from build123d import *

# Parameters (mm, degrees)
SKETCH1_R           = 40.52203667
BOSS_EXTRUDE1_DEPTH = 20
FILLET1_R           = 45


with BuildPart() as part:
    # Sketch1 → Boss-Extrude1 (new body)
    with BuildSketch(Plane.XY):
        Polygon((-324.500042801, 0), (-36.61106831, 0), (-36.61106831, -72.630227613), (19.444444444, -30.98937664), (19.444444444, 0), (19.444444444, 300), (-180.555555556, 600), (-380.555555556, 300), (-380.555555556, 0), (-380.555555556, -30.98937664), (-324.500042801, -72.630227613), align=None)
        with Locations((-180.555555556, 199.47796333)):
            Circle(SKETCH1_R, mode=Mode.SUBTRACT)
        Polygon((-350.555555556, 98.955926659), (-307.046121917, 98.955926659), (-350.555555556, 40.384990781), align=None, mode=Mode.SUBTRACT)
        Polygon((-218.052993309, 18.381237109), (-277.907920592, 98.955926659), (-83.203190519, 98.955926659), (-143.058117802, 18.381237109), align=None, mode=Mode.SUBTRACT)
        Polygon((-40.212760909, 30), (-97.055418804, 30), (-68.634089856, 68.259836918), align=None, mode=Mode.SUBTRACT)
        Polygon((-350.555555556, 128.955926659), (-307.046121917, 128.955926659), (-307.046121917, 178.791030317), (-307.046121917, 221.457829656), (-307.046121917, 270), (-350.555555556, 270), (-350.555555556, 221.457829656), (-350.555555556, 178.791030317), align=None, mode=Mode.SUBTRACT)
        Polygon((-194.895952536, 524.406135398), (-246.308768225, 447.286911864), (-194.895952536, 447.286911864), align=None, mode=Mode.SUBTRACT)
        Polygon((-36.61106831, 330), (-96.633315679, 420.033371054), (-153.463987032, 330), align=None, mode=Mode.SUBTRACT)
        Polygon((-324.500042801, 330), (-207.64712408, 330), (-264.477795432, 420.033371054), align=None, mode=Mode.SUBTRACT)
        Polygon((-10.555555556, 40.384990781), (-54.064989194, 98.955926659), (-10.555555556, 98.955926659), align=None, mode=Mode.SUBTRACT)
        Polygon((-10.555555556, 128.955926659), (-10.555555556, 178.791030317), (-10.555555556, 221.457829656), (-10.555555556, 270), (-54.064989194, 270), (-54.064989194, 221.457829656), (-54.064989194, 178.791030317), (-54.064989194, 128.955926659), align=None, mode=Mode.SUBTRACT)
        Polygon((-320.898350202, 30), (-264.055692307, 30), (-292.477021255, 68.259836918), align=None, mode=Mode.SUBTRACT)
        with BuildLine():
            Line((-279.511482215, 270), (-279.511482215, 221.457829656))
            Line((-279.511482215, 221.457829656), (-247.564832021, 221.457829656))
            ThreePointArc((-247.564832021, 221.457829656), (-232.312774166, 247.379403578), (-207.64712408, 264.58867344))
            Line((-207.64712408, 264.58867344), (-207.64712408, 270))
            Line((-207.64712408, 270), (-279.511482215, 270))
        make_face(mode=Mode.SUBTRACT)
        with BuildLine():
            Line((-279.511482215, 128.955926659), (-279.511482215, 178.791030317))
            Line((-279.511482215, 178.791030317), (-247.975200012, 178.791030317))
            ThreePointArc((-247.975200012, 178.791030317), (-232.771073725, 152.076514844), (-207.64712408, 134.367253219))
            Line((-207.64712408, 134.367253219), (-207.64712408, 128.955926659))
            Line((-207.64712408, 128.955926659), (-279.511482215, 128.955926659))
        make_face(mode=Mode.SUBTRACT)
        with BuildLine():
            Line((-153.463987032, 134.367253219), (-153.463987032, 128.955926659))
            Line((-153.463987032, 128.955926659), (-81.599628896, 128.955926659))
            Line((-81.599628896, 128.955926659), (-81.599628896, 178.791030317))
            Line((-81.599628896, 178.791030317), (-113.135911099, 178.791030317))
            ThreePointArc((-113.135911099, 178.791030317), (-128.340037386, 152.076514844), (-153.463987032, 134.367253219))
        make_face(mode=Mode.SUBTRACT)
        with BuildLine():
            Line((-153.463987032, 264.58867344), (-153.463987032, 270))
            Line((-153.463987032, 270), (-81.599628896, 270))
            Line((-81.599628896, 270), (-81.599628896, 221.457829656))
            Line((-81.599628896, 221.457829656), (-113.54627909, 221.457829656))
            ThreePointArc((-113.54627909, 221.457829656), (-128.798336945, 247.379403578), (-153.463987032, 264.58867344))
        make_face(mode=Mode.SUBTRACT)
        Polygon((-114.802342886, 429.992241235), (-166.215158575, 429.992241235), (-166.215158575, 348.542048906), align=None, mode=Mode.SUBTRACT)
        Polygon((-114.802342886, 447.286911864), (-166.215158575, 524.406135398), (-166.215158575, 447.286911864), align=None, mode=Mode.SUBTRACT)
        Polygon((-246.308768225, 429.992241235), (-194.895952536, 348.542048906), (-194.895952536, 429.992241235), align=None, mode=Mode.SUBTRACT)
    extrude(amount=BOSS_EXTRUDE1_DEPTH)

    # Fillet1
    fillet1_edges = [part.edges().sort_by_distance(p)[0] for p in [
        (19.444444444, -30.98937664, 10),
        (-380.555555556, -30.98937664, 10),
        (-380.555555556, 300, 10),
        (-180.555555556, 600, 10),
        (19.444444444, 300, 10),
    ]]
    fillet(fillet1_edges, radius=FILLET1_R)


solid = part.part
CAD build for the part. Positions are in the model's coordinates, mm. A direction names the side the tool comes from. Give positions to 0.01 mm unless a question says otherwise; leave off trailing zeros. Loops run counter-clockwise (first coordinate to the right, second up) from the corner with the lowest first, then second, coordinate; pieces in that order, holes last. Notation, with made-up numbers: M 83,17 L 90,17 A27 ccw 90,54 Z; hole C -17,-2.75 d4. An arc over 180 degrees is marked long. Write each question's results on one line, items separated by ' | '.
Q1. Mould opens along Y. For faces 3 (the face through (-36.611, -36, 10)), 4 (the face through (-181.17, 563.87, 10.14)), 5 (the face through (-140.15, 485.31, 9.86)) say: pulls with the +Y half, pulls with the -Y half, needs draft (parallel to the pull), parting line crosses it, or undercut.
Geometry check:
face 3: needs draft | face 4: pulls with the +Y half | face 5: undercut
Q2. Band-saw the part on D-D on z = 7.5. Give the number of separate pieces and of enclosed holes in the cut face, and give its area (3 significant figures).
Geometry check:
separate pieces: 1 | enclosed holes: 18 | area: 123,000 mm²
Q3. Band-saw the part on B-B on x = -338. Write the cut outline in (y, z).
Geometry check:
outline: M -62.6,0 L 57.29,0 L 57.29,20 L -62.6,20 Z; M 98.96,0 L 128.96,0 L 128.96,20 L 98.96,20 Z; M 270,0 L 363.83,0 L 363.83,20 L 270,20 Z
Q4. Band-saw the part on A-A on y = 209. Write the cut outline in (x, z).
Geometry check:
outline: M -380.56,0 L -350.56,0 L -350.56,20 L -380.56,20 Z; M -307.05,0 L -219.94,0 L -219.94,20 L -307.05,20 Z; M -141.17,0 L -54.06,0 L -54.06,20 L -141.17,20 Z; M -10.56,0 L 19.44,0 L 19.44,20 L -10.56,20 Z
Q5. Flat gauge pins, fed straight in: P1, Ø8, axis at x = -188.5, y = 493.5, coming from the -Z side; P2, Ø10, axis at y = 361.5, z = 9, coming from the -X side; P3, Ø2, axis at x = -224.5, z = 3.5, coming from the +Y side; P4, Ø10, axis at y = 497, z = 10, coming from the -X side. Where does each tip first touch, or does it go through?
Geometry check:
P1: stops at z = 0 | P2: stops at x = -342.89 | P3: stops at y = 535.58 | P4: stops at x = -252.56
Q6. Which spindle directions (+Z, -Z, +X, -X, +Y, -Y) get a long thin tool onto all of the face, cutting with end or side? Do faces 1 (the face through (-380.556, 141, 10)), 2 (the face through (-81.6, 246, 10)). Say none if no direction does.
Geometry check:
face 1: +Z, -Z, -X, +Y, -Y | face 2: +Z, -Z
Q7. Band-saw the part on C-C on y = 372. Write the cut outline in (x, z), and give its area (3 significant figures).
Geometry check:
outline: M -332.56,0 L -296.5,0 L -296.5,20 L -332.56,20 Z; M -234.16,0 L -209.7,0 L -209.7,20 L -234.16,20 Z; M -194.9,0 L -166.22,0 L -166.22,20 L -194.9,20 Z; M -151.41,0 L -126.95,0 L -126.95,20 L -151.41,20 Z; M -64.61,0 L -28.56,0 L -28.56,20 L -64.61,20 Z | area: 2,990 mm²
Q8. Probe probe 1 along Y at (x, z) = (-202, 13.25); probe 2 along X at (y, z) = (512, 19); probe 3 along Y at (x, z) = (-157.5, 16). List the from-to ranges inside material, lowest first.
Geometry check:
probe 1: y = 0 to 18.38, 98.96 to 165.1, 233.86 to 359.8, 429.99 to 447.29, 513.75 to 558.44 | probe 2: x = -239.22 to -203.17, -194.9 to -166.22, -157.94 to -121.89 | probe 3: y = 0 to 18.38, 98.96 to 166.15, 232.8 to 362.35, 429.99 to 447.29, 511.33 to 557.52
